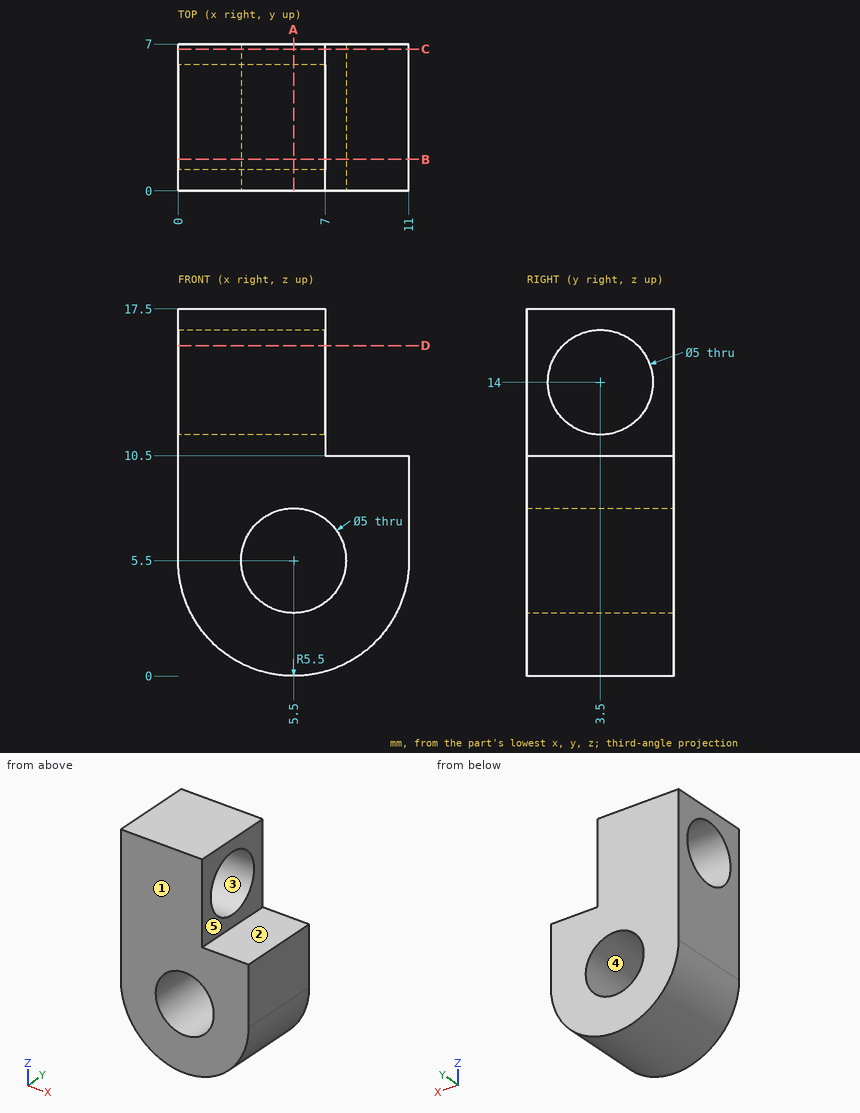
Could you check a few things on this drawing? It's one solid part, dimensions in mm from its lowest x, y, z. A direction names the side the tool comes from. Coordinates: 2 decimals unless noted, no trailing zeros. Order: outer loops, then holes, each group sorted by start corner. A loop starts at its lowest first (then second) coordinate and runs counter-clockwise, first axis right, second up. Notation, with made-up numbers: (28.5, -7.75) -> (45.5, -7.75) arc R24 ccw to (45.5, 12.25) -> close; hole circle Ø7 at (22, 19). An arc over 180 degrees is marked (long way). One line per item, written item: value. Start each with the question number.
1) Imagine slicing it at D-D on z = 15.75. List the corners of the cut face in (x, y) for me.
2) Which directions (+Z, -Z, +X, -X, +Y, -Y) give clear straight access to the entire face, cutting with the end or side of a thin tool? Please do the marked faces 1 and 2.
3) Imagine slicing it at A-A on x = 5.5. List the corners of the cut face in (y, z) for me, plus the area to 3 significant figures.
4) I'm going to push flat-ended pins straight in: pin 1 (5 mm diameter, centred on x = 3, z = 8.5, fed in from -Y); pin 2 (3.5 mm diameter, centred on y = 3.5, z = 13, fed in from +X); pin 3 (3 mm diameter, centred on y = 3.5, z = 14, fed in from +X). Where does each tip first touch, or does it pass through?
5) If I drill on L1, parallel to Z at x = 4, y = 5.75; L2, parallel to Y at x = 5.25, z = 14; L3, parallel to X at y = 4.75, z = 5.5, over which ranges is the centre line in solid material (lowest first)? Write a range as [from, to].
6) We'd pull the mould along X, two halves only. Please class the marked faces 3, 4 and 5: +X half, -X half, draft (parallel to the pull), parting line (faces both ways), or undercut.
7) Imagine slicing it at B-B on y = 1.5. List the corners of the cut face in (x, z) for me.
8) Imagine slicing it at C-C on y = 6.75. List the corners of the cut face in (x, z) for me, plus the area to 3 significant figures.
Answer list:
1. outline: (0, 0) -> (7, 0) -> (7, 1.71) -> (0, 1.71) -> close; (0, 5.29) -> (7, 5.29) -> (7, 7) -> (0, 7) -> close
2. face 1: +Z, -Z, +X, -X, -Y
2. face 2: +Z, +X, +Y, -Y
3. outline: (0, 0) -> (7, 0) -> (7, 3) -> (0, 3) -> close; (0, 8) -> (7, 8) -> (7, 17.5) -> (0, 17.5) -> close; hole circle Ø5 at (3.5, 14)
3. area: 67.9 mm2
4. pin 1: stops at y = 0
4. pin 2: stops at x = 7
4. pin 3: passes through
5. L1: z = [0.21, 3.5], [7.5, 12.91], [15.09, 17.5]
5. L2: y = [0, 1], [6, 7]
5. L3: x = [0, 3], [8, 11]
6. face 3: draft
6. face 4: undercut
6. face 5: +X half
7. outline: (0, 5.5) arc R5.5 ccw to (11, 5.5) -> (11, 10.5) -> (7, 10.5) -> (7, 12.5) -> (0, 12.5) -> close; (0, 15.5) -> (7, 15.5) -> (7, 17.5) -> (0, 17.5) -> close; hole circle Ø5 at (5.5, 5.5)
8. outline: (0, 5.5) arc R5.5 ccw to (11, 5.5) -> (11, 10.5) -> (7, 10.5) -> (7, 17.5) -> (0, 17.5) -> close; hole circle Ø5 at (5.5, 5.5)
8. area: 132 mm2
